Source: CAD feature listing. Evaluate the final solid. Frame: model axes, mm. A direction names the side the tool comes from. Round coordinates to 2 decimals unless told otherwise and drop trailing zeros. Write each loop counter-clockwise with the first axis right and the second up, starting at its lowest first coordinate (ties: lowest second). Pieces come first, ordered by that corner, then holes.
from build123d import *

# Parameters (mm, degrees)
P_IDAT_VYSUNUT_M1_DEPTH       = 2
VYSUNOUT_TENKOST_NN_2_DEPTH   = 2
SKICA4_R                      = 4.9
P_IDAT_VYSUNUT_M2_DEPTH       = 65
SKICA5_R                      = 1
ODEBRAT_VYSUNUT_M1_DEPTH      = 5
P_IDAT_VYSUNUT_M3_DEPTH       = 2
P_IDAT_VYSUNUT_M4_DEPTH       = 2
ODEBRAT_VYSUNUT_M2_DEPTH      = 94.281831028
ODEBRAT_VYSUNUT_M2_DEPTH_BACK = 94.281831028
SKICA8_OUTSIDE_W              = 95.448
SKICA8_OUTSIDE_H              = 89.948
SKICA8_OUTSIDE_W_2            = 9.9
SKICA8_OUTSIDE_H_2            = 65


# Read off the part's stored shape, not the designer's step: Rozdělit1
with BuildPart() as part:
    # Skica1 → Přidat vysunutím1 (new body)
    with BuildSketch(Plane.XY):
        with BuildLine():
            Line((0, 5), (-60, 5))
            Line((-60, 5), (-60, -5))
            Line((-60, -5), (0, -5))
            ThreePointArc((0, -5), (5, 0), (0, 5))
        make_face()
    extrude(amount=P_IDAT_VYSUNUT_M1_DEPTH)

    # Skica3 → Vysunout tenkostěnný2 (add)
    with BuildSketch(Plane.XY):
        with BuildLine():
            Line((-50, -16.5), (-60, -16.5))
            ThreePointArc((-60, -16.5), (-61.5, -15), (-60, -13.5))
            Line((-60, -13.5), (-50, -13.5))
            ThreePointArc((-50, -13.5), (-47.5, -11), (-50, -8.5))
            Line((-50, -8.5), (-60, -8.5))
            ThreePointArc((-60, -8.5), (-61.5, -7), (-60, -5.5))
            Line((-60, -5.5), (-50, -5.5))
            Line((-50, -5.5), (-50, -4.5))
            Line((-50, -4.5), (-60, -4.5))
            ThreePointArc((-60, -4.5), (-62.5, -7), (-60, -9.5))
            Line((-60, -9.5), (-50, -9.5))
            ThreePointArc((-50, -9.5), (-48.5, -11), (-50, -12.5))
            Line((-50, -12.5), (-60, -12.5))
            ThreePointArc((-60, -12.5), (-62.5, -15), (-60, -17.5))
            Line((-60, -17.5), (-50, -17.5))
            Line((-50, -17.5), (-50, -16.5))
        make_face()
    extrude(amount=VYSUNOUT_TENKOST_NN_2_DEPTH)


with BuildPart() as body_2:
    # Rozdělit1: the piece on the far side of the plane
    add(part.part)
    split(bisect_by=Plane(origin=(0, 0, 0), x_dir=(1, 0, 0), z_dir=(0, 1, 0)), keep=Keep.BOTTOM)

    # Zrcadlit3: body 2 across plane


with BuildPart() as part_1:
    add(part.part)

    # Rozdělit1
    split(bisect_by=Plane(origin=(0, 0, 0), x_dir=(1, 0, 0), z_dir=(0, 1, 0)), keep=Keep.TOP)


with BuildPart() as body_2_1:
    add(body_2.part)
    add(body_2.part.mirror(Plane.ZX))

    # Skica4 → Přidat vysunutím2 (add)
    with BuildSketch(Plane.XY.offset(2)):
        Circle(SKICA4_R)
    extrude(amount=P_IDAT_VYSUNUT_M2_DEPTH)

    # Skica5 → Odebrat vysunutím1 (cut)
    with BuildSketch(Plane.XY.offset(67)):
        Circle(SKICA5_R)
    extrude(amount=-ODEBRAT_VYSUNUT_M1_DEPTH, mode=Mode.SUBTRACT)

    # Skica6 → Přidat vysunutím3 (add)
    with BuildSketch(Plane(origin=(0, 0, 0), x_dir=(-1, 0, 0), z_dir=(0, 0, -1))):
        with BuildLine():
            Line((0, 5), (-5, 5))
            ThreePointArc((-5, 5), (-10, 0), (-5, -5))
            Line((-5, -5), (0, -5))
            ThreePointArc((0, -5), (-5, 0), (0, 5))
        make_face()
    extrude(amount=-P_IDAT_VYSUNUT_M3_DEPTH)

    # Skica7 → Přidat vysunutím4 (add)
    with BuildSketch(Plane.XY.offset(2)):
        with BuildLine():
            Line((-50, 5), (-50, -5))
            Line((-50, -5), (-50, -5.5))
            Line((-50, -5.5), (-60, -5.5))
            ThreePointArc((-60, -5.5), (-61.5, -7), (-60, -8.5))
            Line((-60, -8.5), (-50, -8.5))
            ThreePointArc((-50, -8.5), (-47.5, -11), (-50, -13.5))
            Line((-50, -13.5), (-60, -13.5))
            ThreePointArc((-60, -13.5), (-61.5, -15), (-60, -16.5))
            Line((-60, -16.5), (-50, -16.5))
            Line((-50, -16.5), (-50, -17.5))
            Line((-50, -17.5), (-60, -17.5))
            ThreePointArc((-60, -17.5), (-62.5, -15), (-60, -12.5))
            Line((-60, -12.5), (-50, -12.5))
            ThreePointArc((-50, -12.5), (-48.5, -11), (-50, -9.5))
            Line((-50, -9.5), (-60, -9.5))
            ThreePointArc((-60, -9.5), (-62.5, -7), (-60, -4.5))
            Line((-60, -4.5), (-60, 4.5))
            ThreePointArc((-60, 4.5), (-62.5, 7), (-60, 9.5))
            Line((-60, 9.5), (-50, 9.5))
            ThreePointArc((-50, 9.5), (-48.5, 11), (-50, 12.5))
            Line((-50, 12.5), (-60, 12.5))
            ThreePointArc((-60, 12.5), (-62.5, 15), (-60, 17.5))
            Line((-60, 17.5), (-50, 17.5))
            Line((-50, 17.5), (-50, 16.5))
            Line((-50, 16.5), (-60, 16.5))
            ThreePointArc((-60, 16.5), (-61.5, 15), (-60, 13.5))
            Line((-60, 13.5), (-50, 13.5))
            ThreePointArc((-50, 13.5), (-47.5, 11), (-50, 8.5))
            Line((-50, 8.5), (-60, 8.5))
            ThreePointArc((-60, 8.5), (-61.5, 7), (-60, 5.5))
            Line((-60, 5.5), (-50, 5.5))
            Line((-50, 5.5), (-50, 5))
        make_face()
    extrude(amount=P_IDAT_VYSUNUT_M4_DEPTH)

    # Skica8 outside → Odebrat vysunutím2 (cut, two sides: drawn at the far end of the back side and taken through both)
    with BuildSketch(Plane(origin=(0, 0, 0), x_dir=(1, 0, 0), z_dir=(0, 1, 0)).offset(-ODEBRAT_VYSUNUT_M2_DEPTH_BACK)):
        with Locations((-26.25, -33.5)):
            Rectangle(SKICA8_OUTSIDE_W, SKICA8_OUTSIDE_H)
        with Locations((0.05, -34.5)):
            Rectangle(SKICA8_OUTSIDE_W_2, SKICA8_OUTSIDE_H_2, mode=Mode.SUBTRACT)
    extrude(amount=ODEBRAT_VYSUNUT_M2_DEPTH + ODEBRAT_VYSUNUT_M2_DEPTH_BACK, mode=Mode.SUBTRACT)


solid = body_2_1.part
1) Pull-direction query (Y, two-part tool) for faces 3 (the face through (0, 0, 62)), 4 (the face through (-1.062, -4.783, 34.045)), 5 (the face through (0, 0, 2)); classes: released by +Y, released by -Y, zero draft, split by the parting line, or undercut.
Taken from the geometry:
face 3: undercut
face 4: split by the parting line
face 5: zero draft
2) Material intervals for line 1 (Y direction, x = 0, z = 65.6); line 2 (X direction, y = -0.25, z = 12); line 3 (Z direction, x = 0, y = 0), sorted ascending.
Taken from the geometry:
line 1: y = -4.9 to -1, 1 to 4.9
line 2: x = -4.89 to 4.89
line 3: z = 2 to 62
3) Reachability of faces 1 (the face through (0, -1, 65)), 2 (the face through (-0.1, 1.2, 67)) from +Z, -Z, +X, -X, +Y, -Y: full face, straight path, thin tool, end or side. Return the list, or none.
Taken from the geometry:
face 1: +Z
face 2: +Z, +X, -X, +Y, -Y
4) Section query C-C on z = 12. Return the cut outline in (x, y).
Taken from the geometry:
outline: circle Ø9.8 at (0, 0)
5) Section query D-D on x = 2.75. Return the cut outline in (y, z).
Taken from the geometry:
outline: (-4.06, 2) - (4.06, 2) - (4.06, 67) - (-4.06, 67) - close
6) Contact query for flat-ended pins moving along their axis: P1, Ø1.6, axis at x = 0, y = 0, coming from the +Z side; P2, Ø3, axis at y = 3.5, z = 59.5, coming from the -X side; P3, Ø3, axis at y = 3.5, z = 20, coming from the +X side. Output: stop coordinate, or through.
Taken from the geometry:
P1: stops at z = 62
P2: stops at x = -4.47
P3: stops at x = 4.47
7) Section query A-A on x = 0. Return the cut outline in (y, z).
Taken from the geometry:
outline: (-4.9, 2) - (4.9, 2) - (4.9, 67) - (1, 67) - (1, 62) - (-1, 62) - (-1, 67) - (-4.9, 67) - close
